Input: part model. Units: mm. Frame: model coordinates. A direction names the side the tool comes from. Round coordinates to 2 decimals unless told otherwise and drop trailing zeros. Order: outer loops, then holes, each group sorted by start corner. A loop starts at its lowest first (then second) coordinate and runs counter-clockwise, first axis right, second up. Notation, with made-up numbers: (66.5, -30) -> (122.5, -30) arc R20 ccw to (122.5, -18) -> close; hole circle Ø6 at (74, 41). An arc over 180 degrees is marked (long way). Answer as CSV lines item,"result". Start each with the question number.
1) Line query: L1, parallel to Y at x = 4.5, z = 0.75; L2, parallel to Y at x = -5.08, z = 0.95; L3, parallel to Y at x = -5.25, z = 0.4. Output: solid intervals per line, ascending.
2) Section query B-B, the plane z = 0.35. Output: boundary loops of the cut face in (x, y).
3) First-contact query: P1, Ø4, axis at x = 1.5, y = -2.5, coming from the +Z side; P2, Ø1, axis at y = 2, z = 2.5, coming from the -X side; P3, Ø1.4, axis at x = 0.5, z = 2.5, coming from the -Y side. Flat tips, straight axial feed; report the tip coordinate or a pass-through.
4) Section query A-A, the plane x = 0. Output: boundary loops of the cut face in (y, z).
5) Mould query, pull axis X, two halves, no side actions, for faces 1 (the face through (2.771, -8.694, 0.789)), 2 (the face through (-1.25, 2, 2)), 3 (the face through (0, 0, 1.6)), 4 (the face through (1.25, 2, 2)). Classes: +X half, -X half, draft (parallel to the pull), parting line (faces both ways), or undercut.
6) Section query C-C, the plane x = 2.54. Output: boundary loops of the cut face in (y, z), and give its area (3 significant figures).
7) Section query D-D, the plane x = 5.08. Output: boundary loops of the cut face in (y, z), and give its area (3 significant figures).
8) Access query for faces 5 (the face through (0, 2.7, 2)), 6 (the face through (0, 2, 2.9)), 7 (the face through (0, 1.15, 2)). Directions: +Z, -Z, +X, -X, +Y, -Y. A direction counts if a zero-diameter tool reaches every point of the face in a straight line with its end or side. Return the directions, or none.
```python
from build123d import *

# Parameters (mm, degrees)
F0_W     = 14.1
F0_H     = 18.7
F0_R     = 0.5
F0_R_2   = 1.4
F1_DEPTH = 1.6
F2_W     = 2.5
F2_H     = 1.55
F3_DEPTH = 1.3


with BuildPart() as f1:
    # F0 (on Top) → F1 (new body)
    with BuildSketch(Plane.XY):
        Rectangle(F0_W, F0_H)
        with Locations((-5.08, -8.25)):
            Circle(F0_R, mode=Mode.SUBTRACT)
        with Locations((-2.54, -8.25)):
            Circle(F0_R, mode=Mode.SUBTRACT)
        with Locations((0, -8.25)):
            Circle(F0_R, mode=Mode.SUBTRACT)
        with Locations((2.54, -8.25)):
            Circle(F0_R, mode=Mode.SUBTRACT)
        with Locations((5.08, -8.25)):
            Circle(F0_R, mode=Mode.SUBTRACT)
        with Locations((-4.5, 6.8)):
            Circle(F0_R_2, mode=Mode.SUBTRACT)
        with Locations((4.5, 6.8)):
            Circle(F0_R_2, mode=Mode.SUBTRACT)
    extrude(amount=F1_DEPTH)

    # F2 (on face) → F3 (join)
    with BuildSketch(Plane.XY.offset(1.6)):
        with Locations((0, 1.925)):
            Rectangle(F2_W, F2_H)
    extrude(amount=F3_DEPTH)


solid = f1.part
```
Findings:
1,L1,"y = -9.35 to 5.4, 8.2 to 9.35"
1,L2,"y = -9.35 to -8.75, -7.75 to 5.53, 8.07 to 9.35"
1,L3,"y = -9.35 to -8.72, -7.78 to 5.62, 7.98 to 9.35"
2,outline,"(-7.05, -9.35) -> (7.05, -9.35) -> (7.05, 9.35) -> (-7.05, 9.35) -> close; hole circle Ø2.8 at (-4.5, 6.8); hole circle Ø1 at (-5.08, -8.25); hole circle Ø1 at (-2.54, -8.25); hole circle Ø1 at (0, -8.25); hole circle Ø1 at (2.54, -8.25); hole circle Ø2.8 at (4.5, 6.8); hole circle Ø1 at (5.08, -8.25)"
3,P1,"stops at z = 1.6"
3,P2,"stops at x = -1.25"
3,P3,"stops at y = 1.15"
4,outline,"(-9.35, 0) -> (-8.75, 0) -> (-8.75, 1.6) -> (-9.35, 1.6) -> close; (-7.75, 0) -> (9.35, 0) -> (9.35, 1.6) -> (2.7, 1.6) -> (2.7, 2.9) -> (1.15, 2.9) -> (1.15, 1.6) -> (-7.75, 1.6) -> close"
5,face 1,"undercut"
5,face 2,"-X half"
5,face 3,"draft"
5,face 4,"+X half"
6,outline,"(-9.35, 0) -> (-8.75, 0) -> (-8.75, 1.6) -> (-9.35, 1.6) -> close; (-7.75, 0) -> (9.35, 0) -> (9.35, 1.6) -> (-7.75, 1.6) -> close"
6,area,"28.3 mm^2"
7,outline,"(-9.35, 0) -> (-8.75, 0) -> (-8.75, 1.6) -> (-9.35, 1.6) -> close; (-7.75, 0) -> (5.53, 0) -> (5.53, 1.6) -> (-7.75, 1.6) -> close; (8.07, 0) -> (9.35, 0) -> (9.35, 1.6) -> (8.07, 1.6) -> close"
7,area,"24.2 mm^2"
8,face 5,"+Z, +X, -X, +Y"
8,face 6,"+Z, +X, -X, +Y, -Y"
8,face 7,"+Z, +X, -X, -Y"
